Job drawing, mm, ordinate dimensions from the low corner. One solid piece. A direction names the side the tool comes from. Coordinates: 2 decimals unless noted, no trailing zeros. Order: outer loops, then holes, each group sorted by start corner. A loop starts at its lowest first (then second) coordinate and runs counter-clockwise, first axis right, second up. Notation, with made-up numbers: M -1.75,-8 L 55.25,-8 A10 cw 55.25,-3 Z; hole C 48.25,-21 d7. An arc over 180 degrees is marked long. Write item = value, one per line.
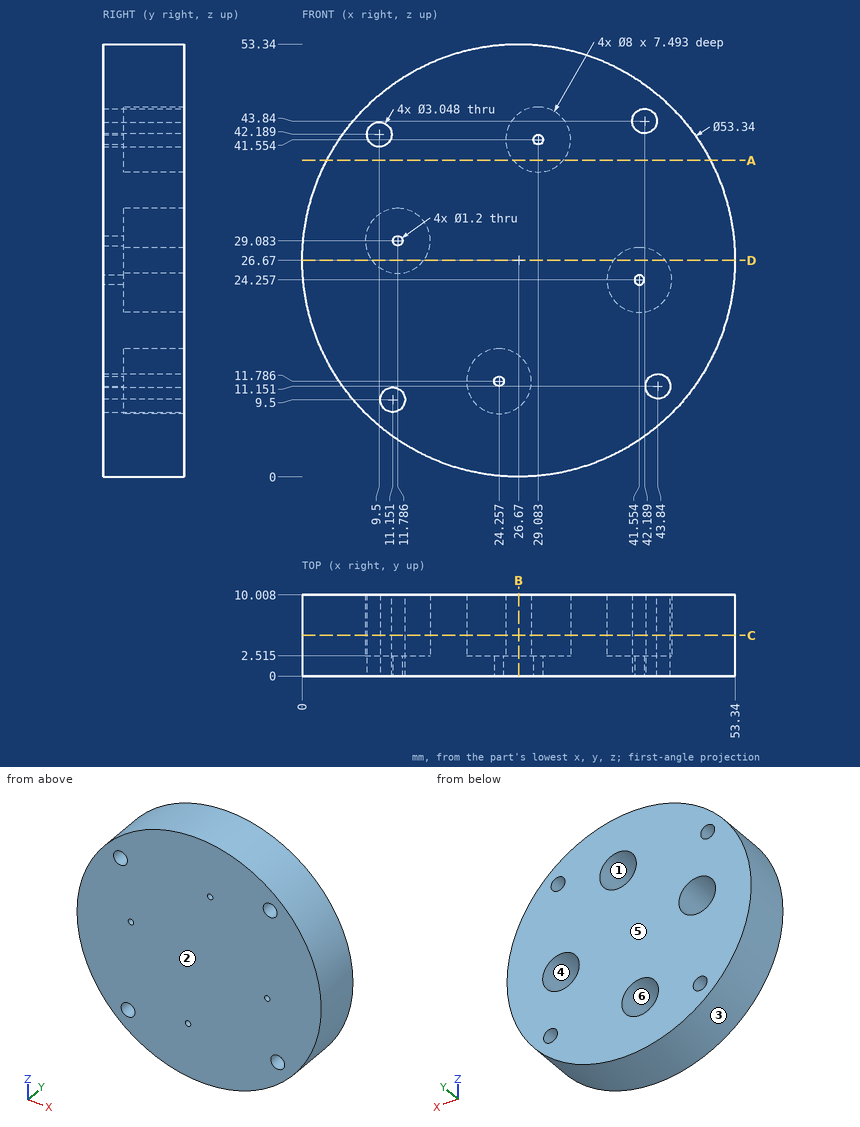
(1) Wall check: line 1 (X direction, y = 0.5, z = 42.5) (1 decimal); line 2 (X direction, y = 2.75, z = 29.5); line 3 (X direction, y = 5.5, z = 14) (1 decimal). Give the ranges that are in metal, low to high. Write a range as from..to.
Evaluation:
line_1 = 5.2..8, 11..41.5, 42.9..48.1
line_2 = 0.15..7.81, 15.76..53.19
line_3 = 3.2..20.9, 27.6..50.1
(2) Pull direction X, two halves, no side cores. Call the marked faces 1, 2, 3 and 4: +X half, -X half, draft (parallel to the pull), parting line (faces both ways), or undercut.
Evaluation:
face_1 = undercut
face_2 = draft
face_3 = parting line
face_4 = undercut
(3) Pin check, flat tips, straight feed: pin 1 Ø2.5 at (x, z) = (43, 26) entering from +Y (1 decimal); pin 2 Ø5 at (x, z) = (43.84, 11.15) entering from +Y; pin 3 Ø6 at (y, z) = (2, 46) entering from +X (1 decimal); pin 4 Ø1.5 at (y, z) = (6.5, 19.5) entering from +X. Stop position of each tip, or through.
Evaluation:
pin_1 = 2.5
pin_2 = 10.01
pin_3 = 47.8
pin_4 = 52.56
(4) Slice it at C-C, the plane y = 5. State how many separate pieces and enclosed holes the cut face has, then the cut area to 3 significant figures.
Evaluation:
separate_pieces = 1
enclosed_holes = 8
area = 2,000 mm²
(5) Slice it at B-B, the plane x = 26.67. Write the cut outline in (y, z) (1 decimal), then the cut area to 3 significant figures.
Evaluation:
outline = M 0,0 L 10,0 L 10,8.6 L 2.5,8.6 L 2.5,15 L 10,15 L 10,38.4 L 2.5,38.4 L 2.5,44.7 L 10,44.7 L 10,53.3 L 0,53.3 Z
area = 438 mm²
(6) Tool access for the marked faces 5 and 6: list every direction of +Z, -Z, +X, -X, +Y, -Y with a clear straight run to the whole face (end or side of a thin tool).
Evaluation:
face_5 = +Z, -Z, +X, -X, +Y
face_6 = +Y
(7) Slice it at A-A, the plane z = 39. Write the cut outline in (x, y) (1 decimal).
Evaluation:
outline = M 3,0 L 50.3,0 L 50.3,10 L 32.2,10 L 32.2,2.5 L 26,2.5 L 26,10 L 3,10 Z
(8) Slice it at D-D, the plane z = 26.67. Write the cut outline in (x, y) (1 decimal).
Evaluation:
outline = M 0,0 L 53.3,0 L 53.3,10 L 44.7,10 L 44.7,2.5 L 38.4,2.5 L 38.4,10 L 15,10 L 15,2.5 L 8.6,2.5 L 8.6,10 L 0,10 Z
